from build123d import *

# Parameters (mm, degrees)
F0_R     = 2.125
F1_DEPTH = 9
F2_T     = -2.5
F3_W     = 9.5
F3_H     = 14
F4_DEPTH = 5.75


with BuildPart() as f1:
    # F0 (on Top) → F1 (new body)
    with BuildSketch(Plane.XY):
        with BuildLine():
            ThreePointArc((32.5, 9), (31.035534, 12.535534), (27.5, 14))
            Line((27.5, 14), (-27.5, 14))
            ThreePointArc((-27.5, 14), (-31.035534, 12.535534), (-32.5, 9))
            Line((-32.5, 9), (-32.5, -9))
            ThreePointArc((-32.5, -9), (-31.035534, -12.535534), (-27.5, -14))
            Line((-27.5, -14), (27.5, -14))
            ThreePointArc((27.5, -14), (31.035534, -12.535534), (32.5, -9))
            Line((32.5, -9), (32.5, 9))
        make_face()
        Circle(F0_R, mode=Mode.SUBTRACT)
    extrude(amount=F1_DEPTH)

    # F2
    f2_openings = [f1.faces().sort_by_distance(p)[0] for p in [
        (30.535084, 12.035084, 9),
    ]]
    offset(amount=F2_T, openings=f2_openings)

    # F3 (on face) → F4 (cut)
    with BuildSketch(Plane.XY.offset(9)):
        with Locations((9.75, 7)):
            Rectangle(F3_W, F3_H)
        with Locations((9.75, -7)):
            Rectangle(F3_W, F3_H)
        with Locations((-9.75, -7)):
            Rectangle(F3_W, F3_H)
        with Locations((-9.75, 7)):
            Rectangle(F3_W, F3_H)
        with Locations((23.25, 7)):
            Rectangle(F3_W, F3_H)
        with Locations((-23.25, 7)):
            Rectangle(F3_W, F3_H)
    extrude(amount=-F4_DEPTH, mode=Mode.SUBTRACT)


solid = f1.part
Read the model definition and answer for the solid it produces. Units are mm, in the model's axes. A direction names the side the tool comes from. Give positions to 0.01 mm unless a question says otherwise; leave off trailing zeros. Loops run counter-clockwise (first coordinate to the right, second up) from the corner with the lowest first, then second, coordinate; pieces in that order, holes last. Notation, with made-up numbers: (-14, 53) -> (6, 53) arc R20 cw to (6, 60) -> close; hole circle Ø5 at (7, 38.5). An arc over 180 degrees is marked (long way). Use a Markdown table: item, result.
Q1. Section B-B, the plane y = 0 is taken. Determine the outline of the cut face in (x, z) (3 decimals), then the cut area to 3 significant figures.
Solved:
| item | result |
|---|---|
| outline | (-32.5, 0) -> (-2.125, 0) -> (-2.125, 9) -> (-4.625, 9) -> (-4.625, 2.5) -> (-30, 2.5) -> (-30, 9) -> (-32.5, 9) -> close; (2.125, 0) -> (32.5, 0) -> (32.5, 9) -> (30, 9) -> (30, 2.5) -> (4.625, 2.5) -> (4.625, 9) -> (2.125, 9) -> close |
| area | 217 mm^2 |
Q2. Each of these flat-tipped pins is pushed along its axis until it touches: pin 1 (0.8 mm diameter, centred on y = 12.5, z = 7.5, fed in from -X); pin 2 (1.2 mm diameter, centred on x = 11, y = 12.5, fed in from +Z); pin 3 (3 mm diameter, centred on y = -13, z = 6, fed in from +X); pin 4 (5 mm diameter, centred on x = 9, z = 6, fed in from -Y). Where does it stop, or does it pass through?
Solved:
| item | result |
|---|---|
| pin 1 | stops at x = -31.42 |
| pin 2 | stops at z = 3.25 |
| pin 3 | stops at x = 31.83 |
| pin 4 | passes through |
Q3. Section C-C, the plane z = 6.75 is taken. Count the separate pieces of the cut face and the enclosed holes in it, then the cut area to 3 significant figures.
Solved:
| item | result |
|---|---|
| separate pieces | 7 |
| enclosed holes | 1 |
| area | 334 mm^2 |
Q4. Section A-A, the plane x = 0 is taken. Determine the outline of the cut face in (y, z) (3 decimals), then the cut area to 3 significant figures.
Solved:
| item | result |
|---|---|
| outline | (-14, 0) -> (-2.125, 0) -> (-2.125, 9) -> (-4.625, 9) -> (-4.625, 2.5) -> (-11.5, 2.5) -> (-11.5, 9) -> (-14, 9) -> close; (2.125, 0) -> (14, 0) -> (14, 9) -> (11.5, 9) -> (11.5, 2.5) -> (4.625, 2.5) -> (4.625, 9) -> (2.125, 9) -> close |
| area | 124 mm^2 |
Q5. A tool of negligible diameter and unlimited length cuts with its end or side. For faces 3 (the face through (0, -11.5, 6)), 4 (the face through (18.5, 13, 6)), 5 (the face through (14.5, -13, 6)), from which of +Z, -Z, +X, -X, +Y, -Y can it reach the whole face along a straight path? Write none if from no direction.
Solved:
| item | result |
|---|---|
| face 3 | +Z |
| face 4 | +Z, +Y |
| face 5 | +Z, +Y, -Y |
Q6. Determine the mould class of faces 1 (the face through (1.142, 1.792, 4.437)), 2 (the face through (5, 13, 6)) for opening direction Y: pulls with the +Y half, pulls with the -Y half, needs draft (parallel to the pull), parting line crosses it, or undercut.
Solved:
| item | result |
|---|---|
| face 1 | undercut |
| face 2 | needs draft |
Q7. Find the intervals of material crossed by line 1 along Y through (x, z) = (0, 4.25) (3 decimals); line 2 along Y through (x, z) = (0, 2) (3 decimals); line 3 along X through (y, z) = (9, 8.5), in increasing order.
Solved:
| item | result |
|---|---|
| line 1 | y = -14 to -11.5, -4.625 to -2.125, 2.125 to 4.625, 11.5 to 14 |
| line 2 | y = -14 to -2.125, 2.125 to 14 |
| line 3 | x = -32.5 to -30, 30 to 32.5 |
Q8. Section D-D, the plane x = -10 is taken. Determine the outline of the cut face in (y, z).
Solved:
| item | result |
|---|---|
| outline | (-14, 0) -> (14, 0) -> (14, 3.25) -> (11.5, 3.25) -> (11.5, 2.5) -> (-11.5, 2.5) -> (-11.5, 3.25) -> (-14, 3.25) -> close |
